Model file for the job. Use its own axes, mm. Coordinates: 2 decimals unless noted, no trailing zeros. Loops run counter-clockwise (first coordinate to the right, second up) from the corner with the lowest first, then second, coordinate; pieces in that order, holes last. Notation, with made-up numbers: (-18.5, 52) - (23.5, 52) arc R10 cw to (23.5, 68) - close; hole circle Ø11 at (69.5, 35.25). An arc over 180 degrees is marked (long way). Write each question's results on one line, items separated by ' | '. Start each with the question number.
```python
from build123d import *

# Parameters (mm, degrees)
SKETCH_1_R          = 4.6
SKETCH_1_R_2        = 2.6
EXTRUDE_1_DEPTH     = 16.5
SKETCH_2_R          = 5.1
SKETCH_2_R_2        = 3.1
EXTRUDE_2_DEPTH     = 23.25
EXTRUDE_3_DEPTH     = 2.5
SKETCH_4_W          = 4
SKETCH_4_H          = 5
EXTRUDE_4_DEPTH     = 14
SKETCH_5_W          = 5
SKETCH_5_H          = 5
EXTRUDE_5_DEPTH     = 21
SKETCH_7_W          = 23.250119988
SKETCH_7_H          = 22.5
SKETCH_7_W_2        = 28.223053091
SKETCH_7_H_2        = 34.5
CUT_EXTRUDE_1_DEPTH = 21
FILLET_1_R          = 2
FILLET_2_R          = 4
FILLET_3_R          = 4


with BuildPart() as part:
    # Sketch 1 → Extrude 1 (new, symmetric)
    with BuildSketch(Plane.XY):
        Circle(SKETCH_1_R)
        Circle(SKETCH_1_R_2, mode=Mode.SUBTRACT)
    extrude(amount=EXTRUDE_1_DEPTH, both=True)



with BuildPart() as body_2:
    # Sketch 2 → Extrude 2 (new, symmetric)
    with BuildSketch(Plane.XY):
        with Locations(Location((135.83, 0, 0), (0, 0, 180))):
            Circle(SKETCH_2_R)
        with Locations(Location((135.83, 0, 0), (0, 0, 180))):
            Circle(SKETCH_2_R_2, mode=Mode.SUBTRACT)
    extrude(amount=EXTRUDE_2_DEPTH, both=True)


with BuildPart() as part_1:
    add(part.part)

    add(body_2.part)  # Extrude 3 merges body 2
    # Sketch 3 → Extrude 3 (add, symmetric)
    with BuildSketch(Plane(origin=(0, 0, 0), x_dir=(1, 0, 0), z_dir=(0, 1, 0))):
        with BuildLine():
            Line((132.183492931, 22.25), (77.939764295, 22.25))
            ThreePointArc((77.939764295, 22.25), (63.354138409, 26.932163446), (49.734070133, 19.920966887))
            Line((49.734070133, 19.920966887), (3.331299064, 15.992872298))
            Line((3.331299064, 15.992872298), (3.668700936, 12.007127702))
            Line((3.668700936, 12.007127702), (47.661946379, 15.731250754))
            Line((47.661946379, 15.731250754), (51.828770684, 16.083981413))
            ThreePointArc((51.828770684, 16.083981413), (63.593703521, 22.938077996), (76.377060253, 18.25))
            Line((76.377060253, 18.25), (81.535945694, 18.25))
            Line((81.535945694, 18.25), (132.183492931, 18.25))
            Line((132.183492931, 18.25), (132.183492931, 22.25))
        make_face()
        with BuildLine():
            Line((132.183492931, -18.25), (81.535945694, -18.25))
            Line((81.535945694, -18.25), (76.377060253, -18.25))
            ThreePointArc((76.377060253, -18.25), (63.593703521, -22.938077996), (51.828770684, -16.083981413))
            Line((51.828770684, -16.083981413), (47.661946379, -15.731250754))
            Line((47.661946379, -15.731250754), (3.668700936, -12.007127702))
            Line((3.668700936, -12.007127702), (3.331299064, -15.992872298))
            Line((3.331299064, -15.992872298), (49.734070133, -19.920966887))
            ThreePointArc((49.734070133, -19.920966887), (63.354138409, -26.932163446), (77.939764295, -22.25))
            Line((77.939764295, -22.25), (132.183492931, -22.25))
            Line((132.183492931, -22.25), (132.183492931, -18.25))
        make_face()
    extrude(amount=EXTRUDE_3_DEPTH, both=True)

    # Sketch 4 → Extrude 4 (add, symmetric)
    with BuildSketch(Plane.XY):
        with Locations((22, 0)):
            Rectangle(SKETCH_4_W, SKETCH_4_H)
    extrude(amount=EXTRUDE_4_DEPTH, both=True)

    # Sketch 5 → Extrude 5 (add, symmetric)
    with BuildSketch(Plane.XY):
        with Locations((113.33, 0)):
            Rectangle(SKETCH_5_W, SKETCH_5_H)
    extrude(amount=EXTRUDE_5_DEPTH, both=True)

    # Sketch 7 → Cut-Extrude 1 (cut, symmetric)
    with BuildSketch(Plane(origin=(0, 0, 0), x_dir=(1, 0, 0), z_dir=(0, 1, 0))):
        Rectangle(SKETCH_7_W, SKETCH_7_H)
        with Locations((131.320513742, 0)):
            Rectangle(SKETCH_7_W_2, SKETCH_7_H_2)
    extrude(amount=CUT_EXTRUDE_1_DEPTH, both=True, mode=Mode.SUBTRACT)

    # Fillet 1
    fillet_1_edges = [part_1.edges().sort_by_distance(p)[0] for p in [
        (115.83, 0, 18.25),
        (110.83, 0, 18.25),
        (110.83, 0, -18.25),
        (115.83, 0, -18.25),
        (24, 0, 13.728215991),
        (20, 0, 13.38960737),
        (20, 0, -13.38960737),
        (24, 0, -13.728215991),
    ]]
    fillet(fillet_1_edges, radius=FILLET_1_R)

    # Fillet 2
    fillet_2_edges = [part_1.edges().sort_by_distance(p)[0] for p in [
        (51.828770684, 0, -16.083981413),
        (76.377060253, 0, -18.25),
        (77.939764295, 0, -22.25),
        (49.734070133, 0, -19.920966887),
        (76.377060253, 0, 18.25),
        (51.828770684, 0, 16.083981413),
        (49.734070133, 0, 19.920966887),
        (77.939764295, 0, 22.25),
    ]]
    fillet(fillet_2_edges, radius=FILLET_2_R)

    # Fillet 3
    fillet_3_edges = [part_1.edges().sort_by_distance(p)[0] for p in [
        (131.384777846, -2.5, -20.25),
        (131.384777846, 2.5, -20.25),
        (131.384777846, -2.5, 20.25),
        (131.384777846, 2.5, 20.25),
        (3.861346915, 2.5, 14.030588795),
        (3.861346915, -2.5, 14.030588795),
        (3.861346915, -2.5, -14.030588795),
        (3.861346915, 2.5, -14.030588795),
    ]]
    fillet(fillet_3_edges, radius=FILLET_3_R)


solid = part_1.part
```
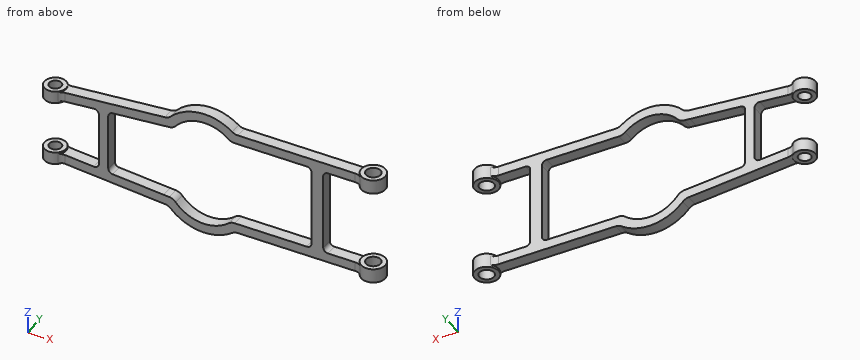
Q1. Cut at D-D (x = 0). List the corners of the cut face in (y, z).
Q2. Pin check, flat tips, straight feed: pin 1 (4 mm diameter, centred on y = 4, z = 2.5, fed in from +X); pin 2 (1 mm diameter, centred on x = 121.5, z = -19.5, fed in from +Y); pin 3 (3 mm diameter, centred on x = 0.5, y = -0.5, fed in from +Z); pin 4 (1.5 mm diameter, centred on y = 1, z = -2, fed in from -X). Stop position of each tip, or through.
Q3. Cut at C-C (y = 0). State how many separate pieces and enclosed holes the cut face has, and give its area (3 significant figures).
Q4. Cut at B-B (z = -0.5). List the corners of the cut face in (x, y).
Q5. Drill centre lines: L1, parallel to X at y = -2, z = -1.5; L2, parallel to Z at x = 134, y = 4; L3, parallel to Z at x = 65, y = 1. Where is each one in solid material? Low to high. Write a range as from..to.
Q6. Cut at A-A (x = 135.83). List the corners of the cut face in (y, z), and give its area (3 significant figures).
Check result:
1) outline: (-4.6, -16.5) - (-2.6, -16.5) - (-2.6, -11.25) - (-4.6, -11.25) - close; (-4.6, 11.25) - (-2.6, 11.25) - (-2.6, 16.5) - (-4.6, 16.5) - close; (2.6, -16.5) - (4.6, -16.5) - (4.6, -11.25) - (2.6, -11.25) - close; (2.6, 11.25) - (4.6, 11.25) - (4.6, 16.5) - (2.6, 16.5) - close
2) pin 1: x = 115.83 | pin 2: y = 2.5 | pin 3: through | pin 4: x = 20
3) separate pieces: 5 | enclosed holes: 1 | area: 1,430 mm²
4) outline: (20, -2.5) - (24, -2.5) - (24, 2.5) - (20, 2.5) - close; (110.83, -2.5) - (115.83, -2.5) - (115.83, 2.5) - (110.83, 2.5) - close
5) L1: 20..24, 110.83..115.83 | L2: -23.25..-17.25, 17.25..23.25 | L3: -27..-23, 23..27
6) outline: (-5.1, -23.25) - (-3.1, -23.25) - (-3.1, -17.25) - (-5.1, -17.25) - close; (-5.1, 17.25) - (-3.1, 17.25) - (-3.1, 23.25) - (-5.1, 23.25) - close; (3.1, -23.25) - (5.1, -23.25) - (5.1, -17.25) - (3.1, -17.25) - close; (3.1, 17.25) - (5.1, 17.25) - (5.1, 23.25) - (3.1, 23.25) - close | area: 48.0 mm²
